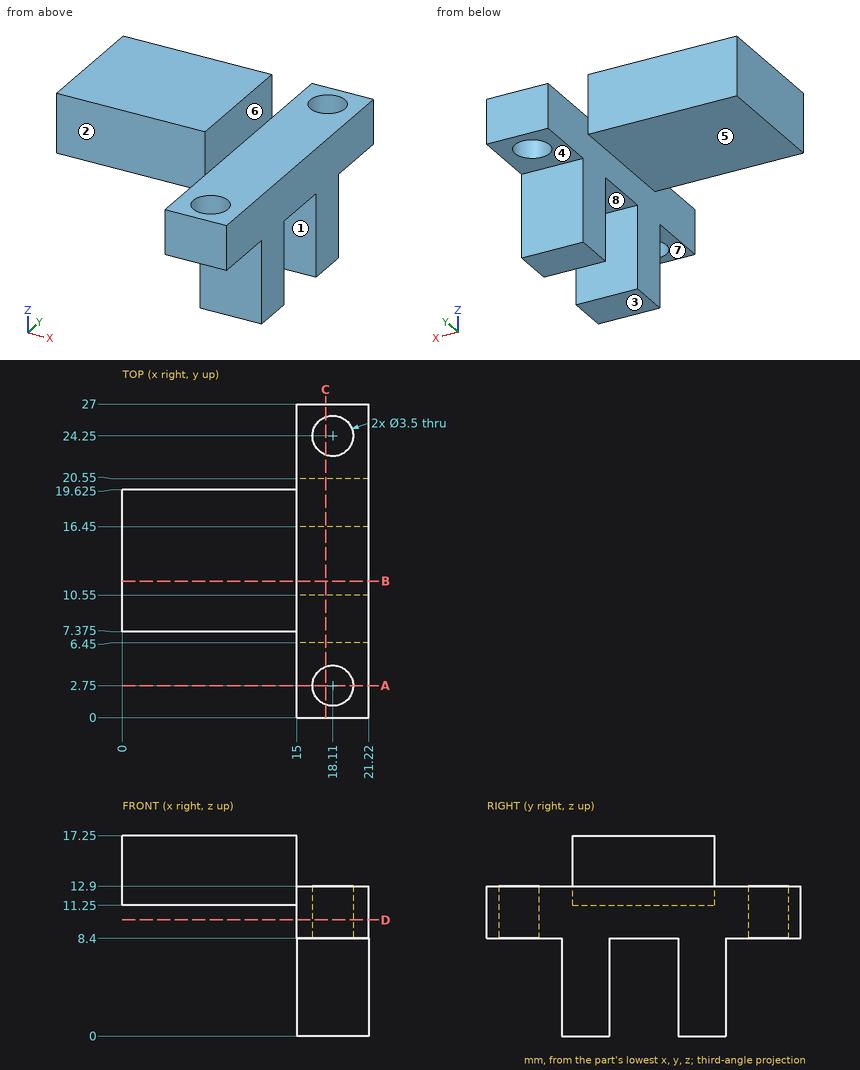
Job drawing, mm, ordinate dimensions from the low corner. One solid piece. A direction names the side the tool comes from. Coordinates: 2 decimals unless noted, no trailing zeros. Order: outer loops, then holes, each group sorted by start corner. A loop starts at its lowest first (then second) coordinate and runs counter-clockwise, first axis right, second up. Notation, with made-up numbers: (-6.75, 78) - (22.25, 78) arc R18 ccw to (22.25, 91) - close; hole circle Ø7 at (-35.75, 52). An arc over 180 degrees is marked (long way). Use CSV: the item, a comma, the result in double quotes.
Item 1: 3-axis set-ups, long thin cutter, end or side, ignore diameter. For the marked faces 4, 5, 6, 7 and 8: which of +Z, -Z, +X, -X, +Y, -Y reach the whole face in a straight line?
Solved:
face 4,"-Z, +X, -X, +Y"
face 5,"-Z, -X, +Y, -Y"
face 6,"+Z, +X, +Y, -Y"
face 7,"-Z, +X, -X, -Y"
face 8,"-Z, +X, -X"
Item 2: Saw through at A-A on y = 2.75. Give the cut face in (x, z).
Solved:
outline,"(15, 8.4) - (16.36, 8.4) - (16.36, 12.9) - (15, 12.9) - close; (19.86, 8.4) - (21.22, 8.4) - (21.22, 12.9) - (19.86, 12.9) - close"
Item 3: Mould opens along Y. For the marked faces 1, 2 and 3 say: +Y half, -Y half, draft (parallel to the pull), parting line (faces both ways), or undercut.
Solved:
face 1,"undercut"
face 2,"-Y half"
face 3,"draft"
Item 4: Saw through at C-C on x = 17.5. Give the cut face in (y, z).
Solved:
outline,"(0, 8.4) - (1.11, 8.4) - (1.11, 12.9) - (0, 12.9) - close; (4.39, 8.4) - (6.45, 8.4) - (6.45, 0) - (10.55, 0) - (10.55, 8.4) - (16.45, 8.4) - (16.45, 0) - (20.55, 0) - (20.55, 8.4) - (22.61, 8.4) - (22.61, 12.9) - (4.39, 12.9) - close; (25.89, 8.4) - (27, 8.4) - (27, 12.9) - (25.89, 12.9) - close"
Item 5: Probe probe 1 along X at (y, z) = (2.75, 10.15); probe 2 along Y at (x, z) = (20, 2); probe 3 along Z at (x, y) = (17, 19.25). List the from-to ranges inside material, lowest first.
Solved:
probe 1,"x = 15 to 16.36, 19.86 to 21.22"
probe 2,"y = 6.45 to 10.55, 16.45 to 20.55"
probe 3,"z = 0 to 12.9"
Item 6: Saw through at B-B on y = 11.75. Give the cut face in (x, z), and give its area (3 significant figures).
Solved:
outline,"(0, 11.25) - (15, 11.25) - (15, 8.4) - (21.22, 8.4) - (21.22, 12.9) - (15, 12.9) - (15, 17.25) - (0, 17.25) - close"
area,"118 mm²"
Item 7: Saw through at D-D on z = 10. Give the cut face in (x, y).
Solved:
outline,"(15, 0) - (21.22, 0) - (21.22, 27) - (15, 27) - close; hole circle Ø3.5 at (18.11, 2.75); hole circle Ø3.5 at (18.11, 24.25)"
Item 8: Drop flat-ended pins along their axis: P1, Ø2, axis at x = 3.5, z = 13.5, coming from the -Y side (3 decimals); P2, Ø4, axis at x = 9, y = 18, coming from the -Z side; P3, Ø1.8, axis at x = 5, z = 13.5, coming from the +Y side (3 decimals). Give the stop position or say it passes through.
Solved:
P1,"stops at y = 7.375"
P2,"stops at z = 11.25"
P3,"stops at y = 19.625"
